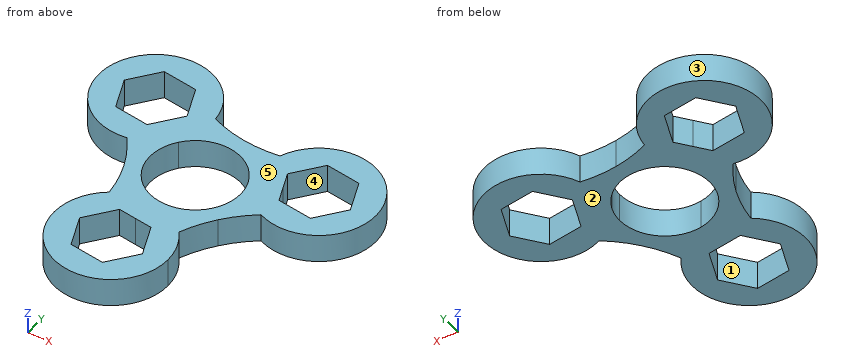
```python
from build123d import *

# Parameters (mm, degrees)
F1_DEPTH = 7


with BuildPart() as f1:
    # F0 (on Top) → F1 (new body)
    with BuildSketch(Plane.XY):
        with BuildLine():
            ThreePointArc((2.1746022478, 14.8415331103), (6.4977862425, 13.5195700356), (10.2307544738, 10.9695789753))
            ThreePointArc((10.2307544738, 10.9695789753), (10.5585141702, 12.900767483), (11.1526052364, 14.7673074037))
            ThreePointArc((11.1526052364, 14.7673074037), (6.6610534474, 14.4959482424), (2.1746022478, 14.8415331103))
        make_face()
        with BuildLine():
            ThreePointArc((-6.6537135081, 13.4435150371), (-2.3461080653, 14.8153898682), (2.1746022478, 14.8415331103))
            ThreePointArc((2.1746022478, 14.8415331103), (-2.222405254, 15.7975651559), (-6.4473076734, 17.3460714654))
            ThreePointArc((-6.4473076734, 17.3460714654), (-6.4074297998, 16.7371058402), (-6.3941287506, 16.1269808862))
            ThreePointArc((-6.3941287506, 16.1269808862), (-6.4591760525, 14.7789848542), (-6.6537135081, 13.4435150371))
        make_face()
        with BuildLine():
            ThreePointArc((-14.6153112984, 3.3753037866), (-16.4516494537, 2.6935577561), (-18.3651659754, 2.2747857513))
            ThreePointArc((-18.3651659754, 2.2747857513), (-15.8843861596, -1.4793326091), (-13.9404458375, -5.5375057427))
            ThreePointArc((-13.9404458375, -5.5375057427), (-14.9571842212, -1.1325370512), (-14.6153112984, 3.3753037866))
        make_face()
        with BuildLine():
            ThreePointArc((-11.7984847082, -14.2565679638), (-10.1191795776, -13.2481782826), (-8.3155687842, -12.484042446))
            ThreePointArc((-8.3155687842, -12.484042446), (-11.6574499679, -9.4394841091), (-13.9404458375, -5.5375057427))
            ThreePointArc((-13.9404458375, -5.5375057427), (-12.5698901189, -9.8234419736), (-11.7984847082, -14.2565679638))
        make_face()
        with BuildLine():
            ThreePointArc((7.2125607389, -17.042093155), (9.2233325136, -13.0166159499), (11.7658431097, -9.3040279405))
            ThreePointArc((11.7658431097, -9.3040279405), (8.4593976642, -12.3870331863), (4.3845568245, -14.3448827619))
            ThreePointArc((4.3845568245, -14.3448827619), (5.8931352835, -15.5943252391), (7.2125607389, -17.042093155))
        make_face()
        with BuildLine():
            ThreePointArc((18.2457923815, -3.0895035015), (16.5328487354, -2.1393774383), (14.9692822923, -0.959472591))
            ThreePointArc((14.9692822923, -0.959472591), (14.0035578894, -5.375906104), (11.7658431097, -9.3040279405))
            ThreePointArc((11.7658431097, -9.3040279405), (14.792295096, -5.9741234333), (18.2457923815, -3.0895035015))
        make_face()
        with BuildLine():
            ThreePointArc((-15.0224460068, 22.9199938039), (-10.9533439645, 19.7969343363), (-6.4473076734, 17.3460714654))
            ThreePointArc((-6.4473076734, 17.3460714654), (-31.3755826932, 24.8107398249), (-18.3651659754, 2.2747857513))
            ThreePointArc((-18.3651659754, 2.2747857513), (-21.7888075854, 6.0944414943), (-25.7658114944, 9.3339679685))
            Line((-25.7658114944, 9.3339679685), (-28.9628918775, 17.3824881445))
            Line((-28.9628918775, 17.3824881445), (-23.5912091337, 24.1755010623))
            Line((-23.5912091337, 24.1755010623), (-15.0224460068, 22.9199938039))
        make_face()
        with BuildLine():
            ThreePointArc((27.3605198922, 1.5498229669), (22.6213200346, -0.4125930385), (18.2457923815, -3.0895035015))
            ThreePointArc((18.2457923815, -3.0895035015), (31.6851726942, -2.2094309865), (38.1634395091, 9.598343143))
            ThreePointArc((38.1634395091, 9.598343143), (26.7948193926, 23.348828222), (11.1526052364, 14.7673074037))
            ThreePointArc((11.1526052364, 14.7673074037), (16.1723449486, 15.82244014), (20.966359126, 17.646863319))
            Line((20.966359126, 17.646863319), (29.5351222529, 16.3913560607))
            Line((29.5351222529, 16.3913560607), (32.732202636, 8.3428358846))
            Line((32.732202636, 8.3428358846), (27.3605198922, 1.5498229669))
        make_face()
        with BuildLine():
            ThreePointArc((10.2306892415, -25.7253240292), (9.454648576, -21.1289233158), (7.2125607389, -17.042093155))
            ThreePointArc((7.2125607389, -17.042093155), (5.6164626368, -21.9168816343), (4.7994523683, -26.9808312875))
            Line((4.7994523683, -26.9808312875), (-0.5722303754, -33.7738442052))
            Line((-0.5722303754, -33.7738442052), (-9.1409935023, -32.5183369469))
            Line((-9.1409935023, -32.5183369469), (-12.3380738854, -24.4698167708))
            ThreePointArc((-12.3380738854, -24.4698167708), (-11.6679760701, -19.3843412978), (-11.7984847082, -14.2565679638))
            ThreePointArc((-11.7984847082, -14.2565679638), (-10.2342765243, -38.1432231127), (10.2306892415, -25.7253240292))
        make_face()
        with BuildLine():
            ThreePointArc((13.9404458706, 5.5375056594), (14.7327303657, 2.818981371), (15, 0))
            ThreePointArc((15, 0), (14.9923186063, -0.4799820909), (14.9692822923, -0.959472591))
            ThreePointArc((14.9692822923, -0.959472591), (16.5328487354, -2.1393774383), (18.2457923815, -3.0895035015))
            ThreePointArc((18.2457923815, -3.0895035015), (22.6213200346, -0.4125930385), (27.3605198922, 1.5498229669))
            Line((27.3605198922, 1.5498229669), (18.7917567653, 2.8053302252))
            Line((18.7917567653, 2.8053302252), (17.1932165738, 6.8295903133))
            Line((17.1932165738, 6.8295903133), (13.9404458706, 5.5375056594))
        make_face()
        with BuildLine():
            ThreePointArc((10.2307544738, 10.9695789753), (12.3870330043, 8.4593979307), (13.9404458706, 5.5375056594))
            Line((13.9404458706, 5.5375056594), (17.1932165738, 6.8295903133))
            Line((17.1932165738, 6.8295903133), (15.5946763822, 10.8538504013))
            Line((15.5946763822, 10.8538504013), (20.966359126, 17.646863319))
            ThreePointArc((20.966359126, 17.646863319), (16.1723449486, 15.82244014), (11.1526052364, 14.7673074037))
            ThreePointArc((11.1526052364, 14.7673074037), (10.5585141702, 12.900767483), (10.2307544738, 10.9695789753))
        make_face()
        with BuildLine():
            ThreePointArc((-11.76584351, 9.3040274344), (-9.4394840743, 11.6574499961), (-6.6537135081, 13.4435150371))
            ThreePointArc((-6.6537135081, 13.4435150371), (-6.4591760525, 14.7789848542), (-6.3941287506, 16.1269808862))
            ThreePointArc((-6.3941287506, 16.1269808862), (-6.4074297998, 16.7371058402), (-6.4473076734, 17.3460714654))
            ThreePointArc((-6.4473076734, 17.3460714654), (-10.9533439645, 19.7969343363), (-15.0224460068, 22.9199938039))
            Line((-15.0224460068, 22.9199938039), (-11.8253656237, 14.8714736279))
            Line((-11.8253656237, 14.8714736279), (-14.5112069956, 11.474967169))
            Line((-14.5112069956, 11.474967169), (-11.76584351, 9.3040274344))
        make_face()
        with BuildLine():
            ThreePointArc((-14.6153112984, 3.3753037866), (-13.5195700109, 6.4977862939), (-11.76584351, 9.3040274344))
            Line((-11.76584351, 9.3040274344), (-14.5112069956, 11.474967169))
            Line((-14.5112069956, 11.474967169), (-17.1970483675, 8.0784607102))
            Line((-17.1970483675, 8.0784607102), (-25.7658114944, 9.3339679685))
            ThreePointArc((-25.7658114944, 9.3339679685), (-21.7888075854, 6.0944414943), (-18.3651659754, 2.2747857513))
            ThreePointArc((-18.3651659754, 2.2747857513), (-16.4516494537, 2.6935577561), (-14.6153112984, 3.3753037866))
        make_face()
        with BuildLine():
            Line((-2.6820095782, -18.3045574823), (-2.1746023607, -14.8415330938))
            ThreePointArc((-2.1746023607, -14.8415330938), (-5.3759058028, -14.003558005), (-8.3155687842, -12.484042446))
            ThreePointArc((-8.3155687842, -12.484042446), (-10.1191795776, -13.2481782826), (-11.7984847082, -14.2565679638))
            ThreePointArc((-11.7984847082, -14.2565679638), (-11.6679760701, -19.3843412978), (-12.3380738854, -24.4698167708))
            Line((-12.3380738854, -24.4698167708), (-6.9663911416, -17.6768038531))
            Line((-6.9663911416, -17.6768038531), (-2.6820095782, -18.3045574823))
        make_face()
        with BuildLine():
            ThreePointArc((7.2125607389, -17.042093155), (5.8931352835, -15.5943252391), (4.3845568245, -14.3448827619))
            ThreePointArc((4.3845568245, -14.3448827619), (1.1325370065, -14.9571842246), (-2.1746023607, -14.8415330938))
            Line((-2.1746023607, -14.8415330938), (-2.6820095782, -18.3045574823))
            Line((-2.6820095782, -18.3045574823), (1.6023719853, -18.9323111115))
            Line((1.6023719853, -18.9323111115), (4.7994523683, -26.9808312875))
            ThreePointArc((4.7994523683, -26.9808312875), (5.6164626368, -21.9168816343), (7.2125607389, -17.042093155))
        make_face()
        with BuildLine():
            ThreePointArc((11.1523566965, 4.4300045275), (10.3004252283, 7.6446709467), (10.2307544738, 10.9695789753))
            ThreePointArc((10.2307544738, 10.9695789753), (6.4977862425, 13.5195700356), (2.1746022478, 14.8415331103))
            ThreePointArc((2.1746022478, 14.8415331103), (-2.3461080653, 14.8153898682), (-6.6537135081, 13.4435150371))
            ThreePointArc((-6.6537135081, 13.4435150371), (-7.674318088, 10.2783556881), (-9.412674808, 7.4432219475))
            Line((-9.412674808, 7.4432219475), (-8.7263339365, 6.9004870138))
            ThreePointArc((-8.7263339365, 6.9004870138), (1.6128300842, 11.0074703779), (10.3391640207, 4.1069833641))
            Line((10.3391640207, 4.1069833641), (11.1523566965, 4.4300045275))
        make_face()
        with BuildLine():
            ThreePointArc((11.7658431097, -9.3040279405), (14.0035578894, -5.375906104), (14.9692822923, -0.959472591))
            ThreePointArc((14.9692822923, -0.959472591), (12.738476179, 1.5069765769), (11.1523566965, 4.4300045275))
            Line((11.1523566965, 4.4300045275), (10.3391640207, 4.1069833641))
            ThreePointArc((10.3391640207, 4.1069833641), (10.9267750213, 2.0907445168), (11.125, 0))
            ThreePointArc((11.125, 0), (7.274025375, -8.4174924914), (-1.6128300842, -11.0074703779))
            Line((-1.6128300842, -11.0074703779), (-1.7396818885, -11.873226475))
            ThreePointArc((-1.7396818885, -11.873226475), (1.4702666292, -12.7427653908), (4.3845568245, -14.3448827619))
            ThreePointArc((4.3845568245, -14.3448827619), (8.4593976642, -12.3870331863), (11.7658431097, -9.3040279405))
        make_face()
        with BuildLine():
            ThreePointArc((-9.412674808, 7.4432219475), (-7.674318088, 10.2783556881), (-6.6537135081, 13.4435150371))
            ThreePointArc((-6.6537135081, 13.4435150371), (-9.4394840743, 11.6574499961), (-11.76584351, 9.3040274344))
            Line((-11.76584351, 9.3040274344), (-9.412674808, 7.4432219475))
        make_face()
        with BuildLine():
            Line((-9.412674808, 7.4432219475), (-11.76584351, 9.3040274344))
            ThreePointArc((-11.76584351, 9.3040274344), (-13.5195700109, 6.4977862939), (-14.6153112984, 3.3753037866))
            ThreePointArc((-14.6153112984, 3.3753037866), (-11.7706918576, 5.0980944442), (-9.412674808, 7.4432219475))
        make_face()
        with BuildLine():
            ThreePointArc((14.9692822923, -0.959472591), (14.9923186063, -0.4799820909), (15, 0))
            ThreePointArc((15, 0), (14.7327303657, 2.818981371), (13.9404458706, 5.5375056594))
            Line((13.9404458706, 5.5375056594), (11.1523566965, 4.4300045275))
            ThreePointArc((11.1523566965, 4.4300045275), (12.738476179, 1.5069765769), (14.9692822923, -0.959472591))
        make_face()
        with BuildLine():
            ThreePointArc((-1.6128300842, -11.0074703779), (-10.3391640207, -4.1069833641), (-8.7263339365, 6.9004870138))
            Line((-8.7263339365, 6.9004870138), (-9.412674808, 7.4432219475))
            ThreePointArc((-9.412674808, 7.4432219475), (-11.7706918576, 5.0980944442), (-14.6153112984, 3.3753037866))
            ThreePointArc((-14.6153112984, 3.3753037866), (-14.9571842212, -1.1325370512), (-13.9404458375, -5.5375057427))
            ThreePointArc((-13.9404458375, -5.5375057427), (-11.6574499679, -9.4394841091), (-8.3155687842, -12.484042446))
            ThreePointArc((-8.3155687842, -12.484042446), (-5.064158091, -11.785332265), (-1.7396818885, -11.873226475))
            Line((-1.7396818885, -11.873226475), (-1.6128300842, -11.0074703779))
        make_face()
        with BuildLine():
            ThreePointArc((-8.3155687842, -12.484042446), (-5.3759058028, -14.003558005), (-2.1746023607, -14.8415330938))
            Line((-2.1746023607, -14.8415330938), (-1.7396818885, -11.873226475))
            ThreePointArc((-1.7396818885, -11.873226475), (-5.064158091, -11.785332265), (-8.3155687842, -12.484042446))
        make_face()
        with BuildLine():
            ThreePointArc((-2.1746023607, -14.8415330938), (1.1325370065, -14.9571842246), (4.3845568245, -14.3448827619))
            ThreePointArc((4.3845568245, -14.3448827619), (1.4702666292, -12.7427653908), (-1.7396818885, -11.873226475))
            Line((-1.7396818885, -11.873226475), (-2.1746023607, -14.8415330938))
        make_face()
        with BuildLine():
            Line((11.1523566965, 4.4300045275), (13.9404458706, 5.5375056594))
            ThreePointArc((13.9404458706, 5.5375056594), (12.3870330043, 8.4593979307), (10.2307544738, 10.9695789753))
            ThreePointArc((10.2307544738, 10.9695789753), (10.3004252283, 7.6446709467), (11.1523566965, 4.4300045275))
        make_face()
    extrude(amount=F1_DEPTH)


solid = f1.part
```
Could you check a few things on this model? Use its own coordinates, in mm. Face numbers are marked on the shaded views. A direction names the side the tool comes from. Coordinates: 2 decimals unless noted, no trailing zeros. Write each loop counter-clockwise with the first axis right and the second up, starting at its lowest first coordinate (ties: lowest second). Pieces come first, ordered by that corner, then holes. Notation, with made-up numbers: (-0.5, 20.25) -> (19.5, 20.25) arc R29 cw to (19.5, 53.25) -> close; hole circle Ø5 at (45, 80). An arc over 180 degrees is marked (long way). One line per question, with ' | ' between items. Start each with the question number.
1. If we section it at B-B (x = -21.5): Please give me the cut outline in (y, z).
2. For the marked faces 4 and 5, which set-ups out of +Z, -Z, +X, -X, +Y, -Y let a thin tool reach every point of the face, with its end or its side?
3. If we section it at D-D (x = -4): Please give me the cut outline in (y, z), and give its area (3 significant figures).
4. If we section it at A-A (y = -28): Please give me the cut outline in (x, z), and give its area (3 significant figures).
5. Thinking about a two-plate mould opening in Y: for the marked faces 1, 2 and 3, which applies, pulls with the +Y half, pulls with the -Y half, needs draft (parallel to the pull), parting line crosses it, or undercut?
6. Will these pins go through, and if not, where does the flat tip stop? P1, Ø1, axis at x = 12.5, z = 2.5, coming from the +Y side; P2, Ø4, axis at x = -15, z = 3, coming from the -Y side; P3, Ø1.5, axis at y = 7.5, z = 5.5, coming from the +X side.
7. Please list where these lines run through material, in increasing order: line 1 along X through (y, z) = (12, 3.25); line 2 along Y through (x, z) = (-0.5, 2.5); line 3 along Y through (x, z) = (0.5, 6.25).
8. If we section it at C-C (y = 12.5): Please give me the cut outline in (x, z), and give its area (3 significant figures).
Return value:
1) outline: (2.17, 0) -> (8.71, 0) -> (8.71, 7) -> (2.17, 7) -> close; (23.87, 0) -> (30.08, 0) -> (30.08, 7) -> (23.87, 7) -> close
2) face 4: +Z, -Z | face 5: +Z, +X, -X, +Y, -Y
3) outline: (-39.72, 0) -> (-33.27, 0) -> (-33.27, 7) -> (-39.72, 7) -> close; (-18.11, 0) -> (-10.38, 0) -> (-10.38, 7) -> (-18.11, 7) -> close; (10.38, 0) -> (16.37, 0) -> (16.37, 7) -> (10.38, 7) -> close | area: 141 mm²
4) outline: (-17.58, 0) -> (-10.94, 0) -> (-10.94, 7) -> (-17.58, 7) -> close; (3.99, 0) -> (10.04, 0) -> (10.04, 7) -> (3.99, 7) -> close | area: 88.9 mm²
5) face 1: undercut | face 2: needs draft | face 3: parting line crosses it
6) P1: stops at y = 18.05 | P2: stops at y = -36.25 | P3: stops at x = 38.1
7) line 1: x = -33.77 to -26.82, -14.1 to 16.5, 31.28 to 37.96 | line 2: y = -39.34 to -33.68, -18.62 to -11.11, 11.11 to 15.35 | line 3: y = -39.06 to -32.42, -18.77 to -11.11, 11.11 to 15.13
8) outline: (-33.92, 0) -> (-27.02, 0) -> (-27.02, 7) -> (-33.92, 7) -> close; (-13.7, 0) -> (16.9, 0) -> (16.9, 7) -> (-13.7, 7) -> close; (31.08, 0) -> (37.86, 0) -> (37.86, 7) -> (31.08, 7) -> close | area: 310 mm²
